Geometry check sheet. Reference: the model listing, model coordinates, mm. A direction names the side the tool comes from. Give positions to 0.01 mm unless a question says otherwise; leave off trailing zeros. Loops run counter-clockwise (first coordinate to the right, second up) from the corner with the lowest first, then second, coordinate; pieces in that order, holes last. Notation, with made-up numbers: (45, 47.5) -> (50, 47.5) arc R9 cw to (50, 63.5) -> close; hole circle Ø2 at (-16.5, 47.5). An arc over 180 degrees is marked (long way). Write item = value, one per line. Start each with the question number.
```python
from build123d import *

# Parameters (mm, degrees)
SKETCH1_W           = 215
SKETCH1_H           = 114
BOSS_EXTRUDE1_DEPTH = 49
SKETCH2_W           = 19
SKETCH2_H           = 110
CUT_EXTRUDE1_DEPTH  = 39
SKETCH3_W           = 15
SKETCH3_H           = 86
BOSS_EXTRUDE3_DEPTH = 18
SKETCH4_R           = 2
CUT_EXTRUDE2_DEPTH  = 8
SKETCH5_R           = 1
CUT_EXTRUDE3_DEPTH  = 2


with BuildPart() as part:
    # Sketch1 → Boss-Extrude1 (new body)
    with BuildSketch(Plane.XY):
        Rectangle(SKETCH1_W, SKETCH1_H)
    extrude(amount=BOSS_EXTRUDE1_DEPTH)

    # Sketch2 → Cut-Extrude1 (cut)
    with BuildSketch(Plane(origin=(0, 0, 0), x_dir=(-1, 0, 0), z_dir=(0, 0, -1))):
        with Locations((-98, 0)):
            Rectangle(SKETCH2_W, SKETCH2_H)
    extrude(amount=-CUT_EXTRUDE1_DEPTH, mode=Mode.SUBTRACT)

    # Sketch3 → Boss-Extrude3 (add)
    with BuildSketch(Plane(origin=(0, 0, 39), x_dir=(-1, 0, 0), z_dir=(0, 0, -1))):
        with Locations((-96, -5)):
            Rectangle(SKETCH3_W, SKETCH3_H)
    extrude(amount=BOSS_EXTRUDE3_DEPTH)

    # Sketch4 → Cut-Extrude2 (cut)
    with BuildSketch(Plane(origin=(0, -55, 0), x_dir=(1, 0, 0), z_dir=(0, 1, 0))):
        with Locations((97.5, -10)):
            Circle(SKETCH4_R)
    extrude(amount=-CUT_EXTRUDE2_DEPTH, mode=Mode.SUBTRACT)

    # Sketch5 → Cut-Extrude3 (cut)
    with BuildSketch(Plane.XY.offset(49)):
        with Locations((75, -22)):
            Circle(SKETCH5_R)
        with Locations((-75, -22)):
            Circle(SKETCH5_R)
    extrude(amount=-CUT_EXTRUDE3_DEPTH, mode=Mode.SUBTRACT)


solid = part.part
```
1) Thickness scan on line 1 (Y direction, x = 75, z = 48.05); line 2 (Z direction, x = 97.5, y = -55.95); line 3 (X direction, y = -55.7, z = 10). Record the ranges inside material, lowest first.
2) Section check D-D (z = 28). Enter the section's corners in (x, y).
3) Section check A-A (x = 97.5). Enter the section's corners in (y, z).
4) Section check C-C (y = -33). Enter the section's corners in (x, z), plus the area to 3 significant figures.
5) Tool access check on faces 1 (the flat face through (-2, 1, 49)), 2 (the flat face through (98, -55, 19)). Record the directions out of +Z, -Z, +X, -X, +Y, -Y that give a thin tool (end or side, any length) a straight path to the whole face; none if there is none.
6) Depth check by flat-ended pin: pin 1 Ø5 at (y, z) = (-45, 30) entering from +X; pin 2 Ø1.2 at (x, y) = (-75, -22) entering from +Z. Enter the tip coordinate at first touch or a pass-through.
7) Draft check along Y on faces 3 (the flat face through (-2, -57, 24)), 4 (the cylindrical face through (99.408, -55.986, 9.399)), 5 (the flat face through (88.5, -1, 15)). Enter one of: released by +Y, released by -Y, zero draft, split by the parting line, or undercut.
8) Section check B-B (z = 10). Enter the section's corners in (x, y).
Check result:
q1.line_1 = -57 to -23, -21 to 57
q1.line_2 = 0 to 8, 12 to 49
q1.line_3 = -107.5 to 95.5, 99.5 to 107.5
q2.outline = (-107.5, -57) -> (107.5, -57) -> (107.5, -55) -> (88.5, -55) -> (88.5, -48) -> (103.5, -48) -> (103.5, 38) -> (88.5, 38) -> (88.5, 55) -> (107.5, 55) -> (107.5, 57) -> (-107.5, 57) -> close
q3.outline = (-57, 0) -> (-55, 0) -> (-55, 8) -> (-57, 8) -> close; (-57, 12) -> (-55, 12) -> (-55, 39) -> (-48, 39) -> (-48, 21) -> (38, 21) -> (38, 39) -> (55, 39) -> (55, 0) -> (57, 0) -> (57, 49) -> (-57, 49) -> close
q4.outline = (-107.5, 0) -> (88.5, 0) -> (88.5, 21) -> (103.5, 21) -> (103.5, 39) -> (107.5, 39) -> (107.5, 49) -> (-107.5, 49) -> close
q4.area = 10,100 mm2
q5.face_1 = +Z, +X, -X, +Y, -Y
q5.face_2 = -Z, +X
q6.pin_1 = 103.5
q6.pin_2 = 47
q7.face_3 = released by -Y
q7.face_4 = zero draft
q7.face_5 = undercut
q8.outline = (-107.5, -57) -> (95.5, -57) -> (95.5, -55) -> (88.5, -55) -> (88.5, 55) -> (107.5, 55) -> (107.5, 57) -> (-107.5, 57) -> close; (99.5, -57) -> (107.5, -57) -> (107.5, -55) -> (99.5, -55) -> close
